Verification items for the finished model (mm, model axes). Face numbers are marked on the shaded views. Round coordinates to 2 decimals unless told otherwise and drop trailing zeros. Order: outer loops, then holes, each group sorted by start corner. A loop starts at its lowest first (then second) coordinate and runs counter-clockwise, first axis right, second up. Notation, with made-up numbers: M -31,50.25 L 22,50.25 A26 cw 22,77.25 Z; hole C 45.25,-31 d6. An arc over 180 degrees is marked long. Use CSV: the item, a comma, the result in double quotes. Start each with the question number.
Q1. Sectioned sample at A-A (x = 11.5). Enter the section's corners in (y, z), and give its area (3 significant figures).
Q2. Sectioned sample at B-B (y = -4.5). Enter the section's corners in (x, z).
Q3. Sectioned sample at C-C (x = -79). Enter the section's corners in (y, z).
Q4. Gauge pin test, flat ends, axial feed: pin 1 Ø0.8 at (y, z) = (29.5, -2) entering from +X; pin 2 Ø4 at (y, z) = (-36, 2) entering from -X; pin 3 Ø0.9 at (x, y) = (62.5, -30) entering from -Z. Record the tip position at first contact, or that the pin passes through.
Q5. Mould release check, pull along Y, two halves, no side actions. Record for the marked faces 1 and 2: +Y half, -Y half, draft (parallel to the pull), parting line (faces both ways), or undercut.
Q6. Scan lines: line 1 (Y direction, x = -63.1, z = -0.45); line 2 (Y direction, x = 34, z = -1.25); line 3 (Z direction, x = 57, y = 43). Record each from-to range of solid material in increasing order.
Autodesk Inventor part; units mm, degrees
ref_plane "YZ Plane" through (0, 0, 0) normal (1, 0, 0) x (0, 1, 0)
ref_plane "XZ Plane" through (0, 0, 0) normal (0, 1, 0) x (-1, 0, 0)
ref_plane "XY Plane" through (0, 0, 0) normal (0, 0, 1) x (1, 0, 0)
sketch "Skizze1" plane through (0, 0, 0) normal (0, 0, 1) x (1, 0, 0)
  line L0 (-83.1, 50.3) -> (83.1, 50.3)
  line L1 (83.1, 50.3) -> (83.1, -50.3)
  line L2 (83.1, -50.3) -> (-83.1, -50.3)
  line L3 (-83.1, -50.3) -> (-83.1, 50.3)
  point P0 (0, 0)
  point P1 (83.1, 0)
  point P2 (0, 50.3)
  dimension "d0" = 166.2
  dimension "d1" = 100.6
extrude "Extrusion1" add sketch "Skizze1" along normal blind 5.26
sketch "Skizze2" plane through (0, 0, 0) normal (0, 0, -1) x (-1, 0, 0)
  line L0 (-83.1, 50.3) -> (-83.1, -50.3)
  line L1 (83.1, -50.3) -> (83.1, 50.3)
  line L2 (83.1, 50.3) -> (-83.1, 50.3)
  line L3 (-70.6, 31.6) -> (-55.6, 31.6)
  line L4 (-55.6, 31.6) -> (-55.6, 39.1)
  line L5 (-55.6, 39.1) -> (-70.6, 39.1)
  line L6 (-70.6, 39.1) -> (-70.6, 31.6)
  line L7 (-70.6, 31.6) -> (-55.6, 39.1) construction
  line L8 (-55.6, 31.6) -> (-70.6, 39.1) construction
  circle A0 centre (-63.1, 35.35) radius 1.5
  line L9 (55.6, 31.6) -> (70.6, 31.6)
  line L10 (70.6, 31.6) -> (70.6, 39.1)
  line L11 (70.6, 39.1) -> (55.6, 39.1)
  line L12 (55.6, 39.1) -> (55.6, 31.6)
  line L13 (55.6, 31.6) -> (70.6, 39.1) construction
  line L14 (70.6, 31.6) -> (55.6, 39.1) construction
  circle A1 centre (63.1, 35.35) radius 1.5
  line L15 (-55.6, -34.05) -> (-55.6, -26.55)
  circle A2 centre (-63.1, -30.3) radius 1.5
  line L16 (-70.6, -34.05) -> (-55.6, -34.05)
  line L17 (-70.6, -34.05) -> (-55.6, -26.55) construction
  line L18 (-55.6, -34.05) -> (-70.6, -26.55) construction
  line L19 (-55.6, -26.55) -> (-70.6, -26.55)
  line L20 (-70.6, -26.55) -> (-70.6, -34.05)
  line L21 (55.6, -26.55) -> (55.6, -34.05)
  circle A3 centre (63.1, -30.3) radius 1.5
  line L22 (70.6, -34.05) -> (70.6, -26.55)
  line L23 (70.6, -26.55) -> (55.6, -26.55)
  line L24 (55.6, -34.05) -> (70.6, -26.55) construction
  line L25 (70.6, -34.05) -> (55.6, -26.55) construction
  line L26 (55.6, -34.05) -> (70.6, -34.05)
  point P0 (0, 0)
  point P1 (63.1, 35.35)
  point P2 (-63.1, -30.3)
  point P3 (63.1, -30.3)
  point P4 (63.1, -30.3)
  dimension "d4" = 20
  dimension "d7" = 126.2
  dimension "d9" = 14.95
  dimension "d10" = 65.65
  dimension "d11" = 15
  dimension "d12" = 7.5
  dimension "d19" = 3
  dimension "d50" = 126.2
  dimension "d57" = 65.65
extrude "Extrusion2" add sketch "Skizze2" along normal blind 2.5
sketch "Skizze3" plane through (0, 0, 0) normal (0, 0, -1) x (-1, 0, 0)
  line L0 (-82.45, 50.3) -> (82.45, 50.3)
  line L1 (82.45, 50.3) -> (82.45, -50.3)
  line L2 (82.45, -50.3) -> (-82.45, -50.3)
  line L3 (-82.45, -50.3) -> (-82.45, 50.3)
  line L4 (-37.75, 22) -> (-30.25, 22)
  line L5 (-30.25, 22) -> (-30.25, 37)
  line L6 (-30.25, 37) -> (-37.75, 37)
  line L7 (-37.75, 37) -> (-37.75, 22)
  line L8 (-37.75, 22) -> (-30.25, 37) construction
  line L9 (-30.25, 22) -> (-37.75, 37) construction
  circle A0 centre (-34, 29.5) radius 1.25
  line L10 (20.25, 22) -> (27.75, 22)
  line L11 (27.75, 22) -> (27.75, 37)
  line L12 (27.75, 37) -> (20.25, 37)
  line L13 (20.25, 37) -> (20.25, 22)
  line L14 (20.25, 22) -> (27.75, 37) construction
  line L15 (27.75, 22) -> (20.25, 37) construction
  circle A1 centre (24, 29.5) radius 1.25
  line L16 (-37.75, -27) -> (-30.25, -27)
  line L17 (-30.25, -27) -> (-30.25, -12)
  line L18 (-30.25, -12) -> (-37.75, -12)
  line L19 (-37.75, -12) -> (-37.75, -27)
  line L20 (-37.75, -27) -> (-30.25, -12) construction
  line L21 (-30.25, -27) -> (-37.75, -12) construction
  circle A2 centre (-34, -19.5) radius 1.25
  line L22 (20.25, -27) -> (27.75, -27)
  line L23 (27.75, -27) -> (27.75, -12)
  line L24 (27.75, -12) -> (20.25, -12)
  line L25 (20.25, -12) -> (20.25, -27)
  line L26 (20.25, -27) -> (27.75, -12) construction
  line L27 (27.75, -27) -> (20.25, -12) construction
  circle A3 centre (24, -19.5) radius 1.25
  point P0 (0, 0)
  point P1 (-82.45, 0)
  point P2 (0, 50.3)
  point P3 (-34, -19.5)
  point P4 (24, -19.5)
  dimension "d25" = 164.9
  dimension "d26" = 100.6
  dimension "d27" = 48.45
  dimension "d28" = 58
  dimension "d29" = 20.8
  dimension "d30" = 49
  dimension "d31" = 7.5
  dimension "d32" = 15
  dimension "d33" = 2.5
  dimension "d64" = 58
  dimension "d67" = 49
extrude "Extrusion3" add sketch "Skizze3" along normal blind 2.5 contours L7 L6 L5 L4 | L13 L12 L11 L10 | L19 L18 L17 L16 | L25 L24 L23 L22
chamfer "Fase1" distance 2.5 angle 45 16 edges at (70.6, 35.35, -2.5) (55.6, 35.35, -2.5) (34, 22, -2.5) (34, 37, -2.5) (70.6, -30.3, -2.5) (55.6, -30.3, -2.5) (-55.6, -30.3, -2.5) (-70.6, -30.3, -2.5) (-70.6, 35.35, -2.5) (-55.6, 35.35, -2.5) (34, -12, -2.5) (34, -27, -2.5) (-24, -12, -2.5) (-24, -27, -2.5) (-24, 22, -2.5) (-24, 37, -2.5)
sketch "Skizze4" plane through (0, 0, 0) normal (0, 0, -1) x (-1, 0, 0)
  line L0 (-50.25, 45.8) -> (50.25, 45.8) construction
  line L1 (-48.75, 44.3) -> (48.75, 44.3)
  line L2 (48.75, 47.3) -> (-48.75, 47.3)
  arc A0 (-48.75, 47.3) -> (-48.75, 44.3) centre (-48.75, 45.8) ccw
  arc A1 (48.75, 44.3) -> (48.75, 47.3) centre (48.75, 45.8) ccw
  line L3 (-83.1, 50.3) -> (-83.1, -50.3)
  line L4 (83.1, 50.3) -> (-83.1, 50.3)
  line L5 (-33.1, -43.8) -> (33.1, -43.8) construction
  line L6 (-31.6, -45.3) -> (31.6, -45.3)
  line L7 (31.6, -42.3) -> (-31.6, -42.3)
  arc A2 (-31.6, -42.3) -> (-31.6, -45.3) centre (-31.6, -43.8) ccw
  arc A3 (31.6, -45.3) -> (31.6, -42.3) centre (31.6, -43.8) ccw
  line L8 (-83.1, -50.3) -> (83.1, -50.3)
  line L9 (83.1, -50.3) -> (83.1, 50.3)
  point P0 (0, 0)
  point P1 (0, 45.8)
  point P2 (0, -43.8)
  dimension "d70" = 100.5
  dimension "d71" = 3
  dimension "d73" = 3
  dimension "d74" = 3
  dimension "d75" = 5
  dimension "d76" = 50
  dimension "d77" = 50
extrude "Extrusion4" add sketch "Skizze4" along normal blind 0.5 contours A0 L2 A1 L1 | A2 L7 A3 L6
sketch "Skizze6" plane through (-83.1, -50.3, 0) normal (-1, 0, 0) x (0, 0, 1)
  line L0 (5.26, 100.6) -> (5.26, 0)
  line L1 (5.26, 99.6) -> (4.56, 99.6)
  line L2 (4.56, 99.6) -> (4.56, 2.5)
  line L3 (4.56, 2.5) -> (5.26, 2.5)
  line L4 (5.26, 2.5) -> (5.26, 99.6)
  line L5 (0, 0) -> (5.26, 0)
  line L6 (0, 100.6) -> (5.26, 100.6)
  point P0 (0, 50.3)
  dimension "d83" = 0.7
  dimension "d84" = 2.5
  dimension "d85" = 1
extrude "Extrusion6" add sketch "Skizze6" along normal blind 9.8
equation "\"d77\" = d76"
properties part number "Display Controller" material "Stahl, galvanisiert"
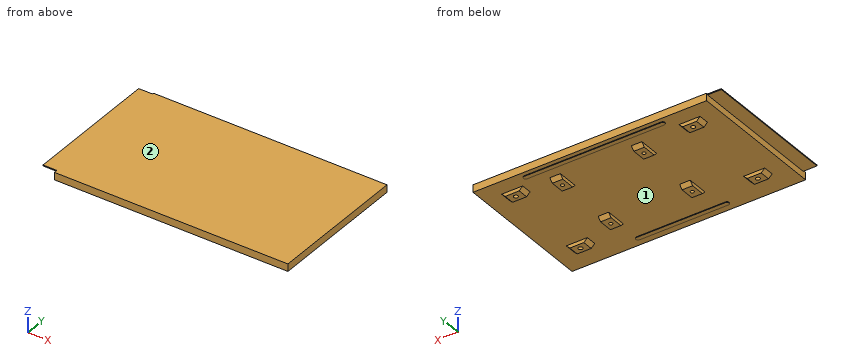
Verdict:
1,outline,"M -50.3,0 L -45.3,0 L -45.3,-0.5 L -42.3,-0.5 L -42.3,0 L 44.3,0 L 44.3,-0.5 L 47.3,-0.5 L 47.3,0 L 50.3,0 L 50.3,5.26 L -50.3,5.26 Z"
1,area,"532 mm²"
2,outline,"M -92.9,4.56 L -83.1,4.56 L -83.1,0 L 83.1,0 L 83.1,5.26 L -92.9,5.26 Z"
3,outline,"M -50.3,0 L 50.3,0 L 50.3,5.26 L -50.3,5.26 Z"
4,pin 1,"stops at x = 37.75"
4,pin 2,"stops at x = -83.1"
4,pin 3,"stops at z = 0"
5,face 1,"undercut"
5,face 2,"draft"
6,line 1,"y = -34.05 to -31.8, -28.8 to -26.55, 31.6 to 33.85, 36.85 to 39.1"
6,line 2,"y = -25.75 to -20.75, -18.25 to -13.25, 23.25 to 28.25, 30.75 to 35.75"
6,line 3,"z = 0 to 5.26"
